Could you check a few things on this model? Use its own coordinates, in mm. Face numbers are marked on the shaded views. Give positions to 0.01 mm unless a question says otherwise; leave off trailing zeros. Loops run counter-clockwise (first coordinate to the right, second up) from the corner with the lowest first, then second, coordinate; pieces in that order, holes last. Notation, with made-up numbers: (39, -17.75) - (45, -17.75) arc R26 ccw to (45, 2.25) - close; hole circle Ø8 at (19.25, 21). An arc over 180 degrees is marked (long way). One line per item, written item: value. Start each with the question number.
Q1. I want a section at B-B (z = 30). Please give me the cut outline in (x, y), then the cut area to 3 significant figures.
Q2. If I drill on line 1 (Z direction, x = 54.5, y = -13); line 2 (Z direction, x = 56, y = -11.75); line 3 (X direction, y = -10.5, z = 5), over which ranges is the centre line in solid material (lowest first)? Write a range as from..to.
Q3. I want a section at D-D (z = 4). Please give me the cut outline in (x, y).
Q4. I want a section at C-C (y = -20). Please give me the cut outline in (x, z).
Q5. I'm going to push a flat-ended pin straight in: P1, Ø4, axis at x = 17.5, z = 6, coming from the -Y side. Where does the tip first touch, or does it pass through?
Q6. If we mould it in two halves opening along Y, with no side actions, what happens to the marked faces 1, 2 and 3? For each: released by +Y, released by -Y, zero draft, split by the parting line, or undercut.
Q7. I want a section at A-A (x = 30). Please give me the cut outline in (y, z).
```python
from build123d import *

# Parameters (mm, degrees)
F0_R     = 2
F0_R_2   = 29
F1_DEPTH = 25


# Not quite as in the source:
# - a feature of the source that left no trace in its solid (it failed there, or was rolled back) is left out


with BuildPart() as f1:
    # F0 (on Front) → F1 (new body)
    with BuildSketch(Plane.XZ):
        with BuildLine():
            ThreePointArc((0, 3), (0.8786796564, 0.8786796564), (3, 0))
            Line((3, 0), (57, 0))
            ThreePointArc((57, 0), (59.1213203436, 0.8786796564), (60, 3))
            Line((60, 3), (60, 57))
            ThreePointArc((60, 57), (59.1213203436, 59.1213203436), (57, 60))
            Line((57, 60), (3, 60))
            ThreePointArc((3, 60), (0.8786796564, 59.1213203436), (0, 57))
            Line((0, 57), (0, 3))
        make_face()
        with Locations((4, 4)):
            Circle(F0_R, mode=Mode.SUBTRACT)
        with Locations((56, 4)):
            Circle(F0_R, mode=Mode.SUBTRACT)
        with Locations((4, 56)):
            Circle(F0_R, mode=Mode.SUBTRACT)
        with Locations((30, 30)):
            Circle(F0_R_2, mode=Mode.SUBTRACT)
        with Locations((56, 56)):
            Circle(F0_R, mode=Mode.SUBTRACT)
    extrude(amount=F1_DEPTH)


solid = f1.part
```
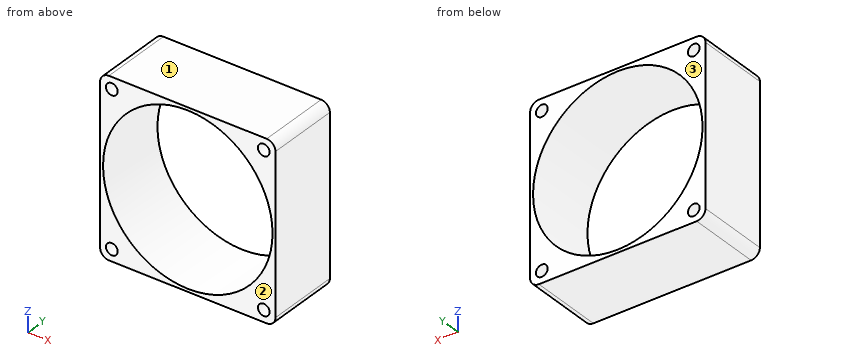
Worked answers:
1. outline: (0, -25) - (1, -25) - (1, 0) - (0, 0) - close; (59, -25) - (60, -25) - (60, 0) - (59, 0) - close
1. area: 50.0 mm²
2. line 1: z = 0..2.68, 5.32..14.48, 45.52..54.68, 57.32..60
2. line 2: z = 0..2, 6..17.15, 42.85..54, 58..60
2. line 3: x = 0..2.27, 5.73..15.3, 44.7..54.27, 57.73..60
3. outline: (0, -25) - (2, -25) - (2, 0) - (0, 0) - close; (6, -25) - (17.15, -25) - (17.15, 0) - (6, 0) - close; (42.85, -25) - (54, -25) - (54, 0) - (42.85, 0) - close; (58, -25) - (60, -25) - (60, 0) - (58, 0) - close
4. outline: (0, 3) arc R3 ccw to (3, 0) - (57, 0) arc R3 ccw to (60, 3) - (60, 57) arc R3 ccw to (57, 60) - (3, 60) arc R3 ccw to (0, 57) - close; hole circle Ø58 at (30, 30); hole circle Ø4 at (4, 4); hole circle Ø4 at (4, 56); hole circle Ø4 at (56, 4); hole circle Ø4 at (56, 56)
5. P1: stops at y = -25
6. face 1: zero draft
6. face 2: released by -Y
6. face 3: released by +Y
7. outline: (-25, 0) - (0, 0) - (0, 1) - (-25, 1) - close; (-25, 59) - (0, 59) - (0, 60) - (-25, 60) - close
